Can you work these out from the model? Positions are in its coordinate system, mm. Coordinates: 2 decimals unless noted, no trailing zeros. Order: outer loops, then holes, each group sorted by start corner. A loop starts at its lowest first (then second) coordinate and runs counter-clockwise, first axis right, second up. Notation, with made-up numbers: (33.5, 67.25) -> (53.5, 67.25) arc R22 ccw to (53.5, 84.25) -> close; hole circle Ø7 at (28.5, 64.25). An arc over 180 degrees is marked (long way). Answer in a Markdown table with one row per item. Add a question column.
1. Will these pins go through, and if not, where does the flat tip stop? pin 1 (3 mm diameter, centred on y = -3.5, z = 11, fed in from +X); pin 2 (5.5 mm diameter, centred on y = -6.35, z = 95.25, fed in from +X); pin 3 (6.5 mm diameter, centred on x = -25, z = 68, fed in from -Y) (3 decimals); pin 4 (4 mm diameter, centred on x = -31.75, y = -8.89, fed in from -Z).
2. Imagine slicing it at B-B on x = -31.75. Write out the boundary of the cut face in (y, z).
3. Imagine slicing it at C-C on z = 37.5. Write out the boundary of the cut face in (x, y) (1 decimal).
4. Imagine slicing it at A-A on x = -10. Write out the boundary of the cut face in (y, z) (3 decimals), plus the area to 3 significant figures.
5. If I drill on line 1 along Z through (x, y) = (-7.5, -6.35) (3 decimals); line 2 along Z through (x, y) = (-30.5, -12); line 3 along Y through (x, z) = (-5.25, 95.25) (3 decimals), over which ranges is the centre line in solid material (lowest first)? Write a range as [from, to].
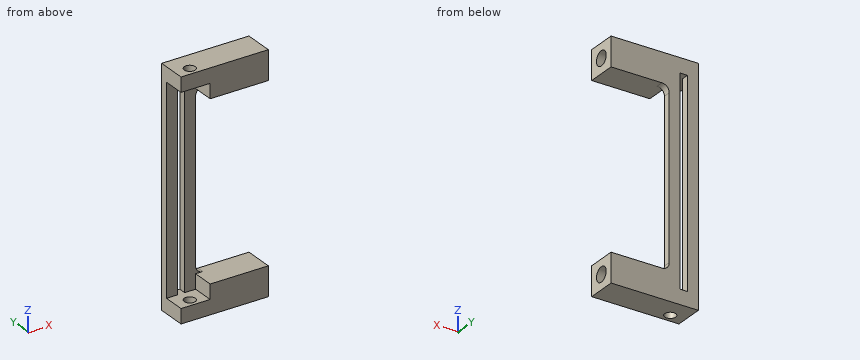
Autodesk Inventor part; units mm, degrees
ref_plane "YZ Plane" through (0, 0, 0) normal (1, 0, 0) x (0, 1, 0)
ref_plane "XZ Plane" through (0, 0, 0) normal (0, 1, 0) x (-1, 0, 0)
ref_plane "XY Plane" through (0, 0, 0) normal (0, 0, 1) x (1, 0, 0)
sketch "Sketch1" plane through (0, 0, 0) normal (0, 1, 0) x (-1, 0, 0)
  line L0 (0, 0) -> (38.1, 0)
  line L1 (38.1, 0) -> (38.1, 12.7)
  line L2 (38.1, 12.7) -> (0, 12.7)
  line L3 (0, 12.7) -> (0, 0)
  dimension "d0" = 38.1
  dimension "d1" = 12.7
sketch "Sketch2" plane through (0, 0, 0) normal (0, 0, 1) x (1, 0, 0)
  line L0 (0, 0) -> (-25.4, 0)
  line L1 (-25.4, 0) -> (-25.4, -12.7)
  line L2 (-25.4, -12.7) -> (0, -12.7)
  line L3 (0, -12.7) -> (0, 0)
  dimension "d2" = 25.4
  dimension "d3" = 12.7
extrude "Extrusion1" add sketch "Sketch2" along normal blind 12.7
sketch "Sketch3" plane through (0, 0, 0) normal (0, 0, -1) x (-1, 0, 0)
  line L0 (0, 0) -> (25.4, 0)
  line L1 (25.4, 0) -> (38.1, 0)
  line L2 (38.1, 0) -> (38.1, -12.7)
  line L3 (38.1, -12.7) -> (25.4, -12.7)
  line L4 (25.4, -12.7) -> (25.4, 0)
  dimension "d6" = 12.7
  dimension "d7" = 12.7
extrude "Extrusion2" add sketch "Sketch3" against normal blind 6.35
sketch "Sketch4" plane through (-25.4, 0, 12.7) normal (0, 1, 0) x (1, 0, 0)
  line L0 (-12.7, 12.7) -> (25.4, 12.7)
  line L1 (0, 12.7) -> (-12.7, 12.7)
  line L2 (-12.7, 12.7) -> (-12.7, -88.9)
  line L3 (-12.7, -88.9) -> (0, -88.9)
  line L4 (0, -88.9) -> (0, 12.7)
  dimension "d10" = 101.6
extrude "Extrusion3" add sketch "Sketch4" against normal blind 3.175
sketch "Sketch5" plane through (-25.4, -3.175, 12.7) normal (0, -1, 0) x (1, 0, 0)
  point P0 (25.4, -12.7)
sketch "Sketch6" plane through (-38.1, 0, 101.6) normal (0, 0, 1) x (1, 0, 0)
  line L0 (12.7, -12.7) -> (38.1, -12.7)
  line L1 (0, 0) -> (38.1, 0)
  line L2 (38.1, 0) -> (38.1, -12.7)
  line L3 (38.1, -12.7) -> (0, -12.7)
  line L4 (0, -12.7) -> (0, 0)
extrude "Extrusion4" add sketch "Sketch6" against normal blind 12.7
sketch "Sketch7" plane through (-38.1, 0, 88.9) normal (0, 0, -1) x (-1, 0, 0)
  line L0 (0, -12.7) -> (0, -3.175)
  line L1 (-12.7, -3.175) -> (0, -3.175)
  line L2 (0, -12.7) -> (-12.7, -12.7)
  line L3 (-12.7, -12.7) -> (-12.7, -3.175)
  line L4 (-12.7, -3.175) -> (0, -3.175)
  line L5 (0, -3.175) -> (0, -12.7)
  point P0 (-38.1, 0)
extrude "Extrusion5" cut sketch "Sketch7" against normal blind 6.35
fillet "Fillet1" radius 3.175 2 edges at (-25.4, -1.5875, 12.7) (-25.4, -1.5875, 88.9)
sketch "Sketch8" plane through (-38.1, -12.7, 101.6) normal (0, 0, 1) x (1, 0, 0)
  point P0 (38.1, 12.7)
  point P1 (6.35, 3.81)
hole "Hole1" at (-31.75, -8.89, 101.6) direction (0, 0, -1) diameter 4.826 depth 107.95 tip angle 118
sketch "Sketch9" plane through (-25.4, -3.175, 12.7) normal (0, -1, 0) x (1, 0, 0)
  line L0 (-12.7, 82.55) -> (0, 82.55)
  line L1 (-4.7625, 82.55) -> (-7.9375, 82.55)
  line L2 (-7.9375, 82.55) -> (-7.9375, -6.35)
  line L3 (-7.9375, -6.35) -> (-4.7625, -6.35)
  line L4 (-4.7625, -6.35) -> (-4.7625, 82.55)
  point P0 (25.4, -12.7)
  point P1 (-6.35, 0)
  dimension "d25" = 3.175
  dimension "d26" = 88.9
extrude "Extrusion6" cut sketch "Sketch9" against normal blind 6.35
sketch "Sketch10" plane through (0, -12.7, 101.6) normal (1, 0, 0) x (0, 0, -1)
  line L0 (95.25, 9.525) -> (95.25, 0)
  point P0 (101.6, 12.7)
  point P1 (6.35, 6.35)
  point P2 (95.25, 6.35)
hole "Hole2" at (0, -6.35, 6.35) at (0, -6.35, 95.25) direction (-1, 0, 0) diameter 6.35 depth 12.7 tip angle 118
properties part number "CarBrake"
Answers follow:
| question | item | result |
|---|---|---|
| 1 | pin 1 | stops at x = 0 |
| 1 | pin 2 | stops at x = -12.96 |
| 1 | pin 3 | stops at y = -3.175 |
| 1 | pin 4 | passes through |
| 2 | outline | (-12.7, 0) -> (-11.3, 0) -> (-11.3, 6.35) -> (-12.7, 6.35) -> close; (-12.7, 95.25) -> (-11.3, 95.25) -> (-11.3, 101.6) -> (-12.7, 101.6) -> close; (-6.48, 0) -> (0, 0) -> (0, 6.35) -> (-6.48, 6.35) -> close; (-6.48, 95.25) -> (0, 95.25) -> (0, 101.6) -> (-6.48, 101.6) -> close |
| 3 | outline | (-38.1, -3.2) -> (-33.3, -3.2) -> (-33.3, 0) -> (-38.1, 0) -> close; (-30.2, -3.2) -> (-25.4, -3.2) -> (-25.4, 0) -> (-30.2, 0) -> close |
| 4 | outline | (-12.7, 0) -> (0, 0) -> (0, 12.7) -> (-12.7, 12.7) -> close; (-12.7, 88.9) -> (0, 88.9) -> (0, 101.6) -> (-12.7, 101.6) -> close; hole circle Ø6.35 at (-6.35, 6.35); hole circle Ø6.35 at (-6.35, 95.25) |
| 4 | area | 259 mm² |
| 5 | line 1 | z = [0, 3.175], [9.525, 12.7], [88.9, 92.075], [98.425, 101.6] |
| 5 | line 2 | z = [0, 6.35], [95.25, 101.6] |
| 5 | line 3 | y = [-12.7, -9.525], [-3.175, 0] |
